Source: CAD feature listing. Evaluate the final solid. Frame: model axes, mm. Face numbers are marked on the shaded views. A direction names the side the tool comes from. Coordinates: 2 decimals unless noted, no trailing zeros. Write each loop counter-clockwise with the first axis right and the second up, starting at its lowest first coordinate (ties: lowest second). Pieces come first, ordered by that corner, then holes. Notation, with made-up numbers: M -34.75,21 L 23.25,21 A17 ccw 23.25,43 Z; hole C 75,63 d10. An arc over 180 degrees is marked long. One line per item, written item: value. Start each with the question number.
Item 1: Cut plane A-A, the plane x = 11.5. Output: boundary loops of the cut face in (y, z).
Item 2: Cut plane B-B, the plane y = 166. Output: boundary loops of the cut face in (x, z).
Item 3: Cut plane C-C, the plane z = 10. Output: boundary loops of the cut face in (x, y), then the cut area to 3 significant figures.
Item 4: Ray query, L1, parallel to Y at x = 9, z = 106; L2, parallel to Z at x = 6.5, y = -2; L3, parallel to Z at x = -1, y = 163. Return the intervals inside material, ascending. Write a range as from..to.
Item 5: Cut plane D-D, the plane y = 102. Output: boundary loops of the cut face in (x, z), then the cut area to 3 significant figures.
Item 6: Set-up query: the marked faces 1, 2 and 3. Return all of +Z, -Z, +X, -X, +Y, -Y with unobstructed straight access to the full face (end or side cutting, diameter ignored); none if empty.
Item 7: Pin query (flat end, axial travel): P1, Ø16.5, axis at y = 162, z = -8, coming from the +X side; P2, Ø12, axis at y = 35.5, z = -7, coming from the +X side; P3, Ø8, axis at y = 26.5, z = 82.5, coming from the +X side; P4, Ø12, axis at y = 52.5, z = -7, coming from the -X side. Return the tip coordinate at first contact, or that it passes through.
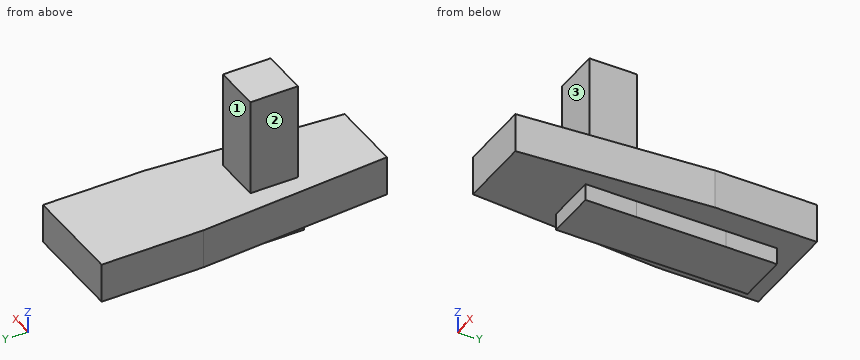
```python
from build123d import *

# Parameters (mm, degrees)
AUFSATZ_LINEAR_AUSTRAGEN1_DEPTH = 35
SKIZZE2_W                       = 42
SKIZZE2_H                       = 42
AUFSATZ_LINEAR_AUSTRAGEN2_DEPTH = 86
SKIZZE3_W                       = 45
SKIZZE3_H                       = 45
AUFSATZ_LINEAR_AUSTRAGEN3_DEPTH = 15


with BuildPart() as part:
    # Skizze1 → Aufsatz-Linear austragen1 (new body)
    with BuildSketch(Plane.XY):
        Polygon((-32.444894928, -45.526866225), (-45, 123.700952226), (-45, 213.700952226), (45, 213.700952226), (45, 123.700952226), (32.555105072, -45.526866225), align=None)
    extrude(amount=AUFSATZ_LINEAR_AUSTRAGEN1_DEPTH)

    # Skizze2 → Aufsatz-Linear austragen2 (add)
    with BuildSketch(Plane.XY.offset(35)):
        with Locations((0, 47.549073259)):
            Rectangle(SKIZZE2_W, SKIZZE2_H)
    extrude(amount=AUFSATZ_LINEAR_AUSTRAGEN2_DEPTH)

    # Skizze3 → Aufsatz-Linear austragen3 (add)
    with BuildSketch(Plane(origin=(0, 0, 0), x_dir=(-1, 0, 0), z_dir=(0, 0, -1))):
        with Locations((0.012439414, 168.70093099)):
            Rectangle(SKIZZE3_W, SKIZZE3_H)
        Polygon((-22.049769251, 67.455627916), (22.950230749, 67.455627916), (22.512439414, 146.20093099), (-22.487560586, 146.20093099), align=None)
        with Locations((0.450230749, 44.955627916)):
            Rectangle(SKIZZE3_W, SKIZZE3_H)
    extrude(amount=AUFSATZ_LINEAR_AUSTRAGEN3_DEPTH)


solid = part.part
```
From the geometry:
1. outline: M -45.53,0 L 22.46,0 L 22.46,-15 L 191.2,-15 L 191.2,0 L 213.7,0 L 213.7,35 L 68.55,35 L 68.55,121 L 26.55,121 L 26.55,35 L -45.53,35 Z
2. outline: M -45,0 L -22.51,0 L -22.51,-15 L 22.49,-15 L 22.49,0 L 45,0 L 45,35 L -45,35 Z
3. outline: M -45,123.7 L -32.44,-45.53 L 32.56,-45.53 L 45,123.7 L 45,213.7 L -45,213.7 Z
3. area: 21,200 mm²
4. L1: y = 26.55..68.55
4. L2: z = 0..35
4. L3: z = -15..35
5. outline: M -43.39,0 L -22.76,0 L -22.76,-15 L 22.24,-15 L 22.24,0 L 43.4,0 L 43.4,35 L -43.39,35 Z
5. area: 3,710 mm²
6. face 1: +Z, +X, -X, +Y
6. face 2: +Z, -X, +Y, -Y
6. face 3: +Z, +X, -X, -Y
7. P1: stops at x = 45
7. P2: stops at x = 22.05
7. P3: stops at x = 21
7. P4: stops at x = -22.95
